Source: three-view drawing plus pictorial views. Frame: mm from the lowest corner of the part. Coordinates: 2 decimals unless noted, no trailing zeros. Order: outer loops, then holes, each group sorted by start corner. A loop starts at its lowest first (then second) coordinate and runs counter-clockwise, first axis right, second up. Notation, with made-up numbers: (89.25, 71.25) - (129.25, 71.25) arc R29 cw to (129.25, 94.25) - close; hole circle Ø8 at (71.25, -38). An arc over 180 degrees is marked (long way). One line per question, with ' | ' between items.
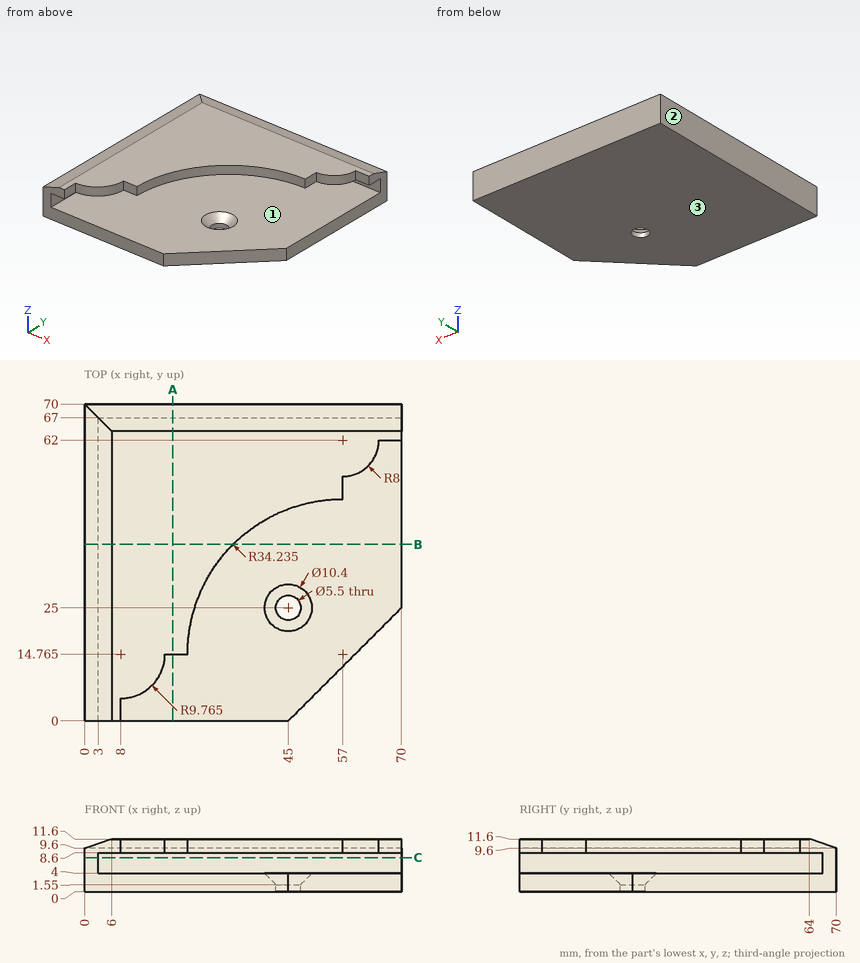
Item 1: Section B-B on y = 39. Return the cut outline in (x, z), and give its area (3 significant figures).
Data:
outline: (0, 0) - (70, 0) - (70, 4) - (3, 4) - (3, 8.6) - (32.82, 8.6) - (32.82, 11.6) - (6, 11.6) - (0, 9.6) - close | area: 386 mm^2
Item 2: Section C-C on z = 7.5. Return the cut outline in (x, y).
Data:
outline: (0, 0) - (3, 0) - (3, 67) - (70, 67) - (70, 70) - (0, 70) - close
Item 3: Ray query, line 1 (Z direction, x = 25, y = 58); line 2 (Z direction, x = 36, y = 38); line 3 (Y direction, x = 11, z = 5). Return the intervals inside material, ascending.
Data:
line 1: 0 to 4, 8.6 to 11.6 | line 2: 0 to 4 | line 3: 67 to 70
Item 4: Contact query for flat-ended pins moving along their axis: P1, Ø1.5, axis at y = 2, z = 10.5, coming from the +X side; P2, Ø0.9, axis at x = 67.5, z = 11, coming from the -Y side; P3, Ø2.5, axis at y = 52.5, z = 11, coming from the +X side. Output: stop coordinate, or through.
Data:
P1: x = 8 | P2: y = 62 | P3: x = 57
Item 5: Draft query along Z for the marked faces 1, 2 and 3. Return one class per face: released by +Z, released by -Z, zero draft, split by the parting line, or undercut.
Data:
face 1: undercut | face 2: zero draft | face 3: released by -Z
Item 6: Section A-A on x = 19.5. Return the cut outline in (y, z) (3 decimals).
Data:
outline: (0, 0) - (70, 0) - (70, 9.6) - (64, 11.6) - (14.765, 11.6) - (14.765, 8.6) - (67, 8.6) - (67, 4) - (0, 4) - close
